Work out the finished part from the listing and answer in its coordinate system (mm). A direction names the side the tool comes from. Give positions to 0.01 mm unless a question says otherwise; leave off trailing zeros. Order: outer loops, then holes, each group sorted by start corner. A loop starts at its lowest first (then second) coordinate and runs counter-clockwise, first axis right, second up. Notation, with made-up numbers: M 67.5,-11.5 L 105.5,-11.5 A6 ccw 105.5,-7.5 Z; hole C 74,75.25 d4. An arc over 180 degrees is marked long. One line per item, written item: value.
from build123d import *

# Parameters (mm, degrees)
F0_R          = 18.15
F0_R_2        = 18.902714
F1_DEPTH      = 76.2
F2_R          = 15.292953
F3_DEPTH      = 38.1
F3_DEPTH_BACK = 38.1


with BuildPart() as f1:
    # F0 (on Front) → F1 (new body)
    with BuildSketch(Plane.XZ):
        with BuildLine():
            Line((35.557076, -57.612903), (35.557076, 57.612903))
            ThreePointArc((35.557076, 57.612903), (0, 93.16998), (-35.557076, 57.612903))
            Line((-35.557076, 57.612903), (-35.557076, -57.612903))
            ThreePointArc((-35.557076, -57.612903), (0, -93.16998), (35.557076, -57.612903))
        make_face()
        with Locations((0, -57.612903)):
            Circle(F0_R, mode=Mode.SUBTRACT)
        with Locations((0, 57.612903)):
            Circle(F0_R_2, mode=Mode.SUBTRACT)
    extrude(amount=F1_DEPTH)

    # F2 (on Top) → F3 (join, two sides)
    with BuildSketch(Plane.XY) as f3_sk:
        with BuildLine():
            ThreePointArc((-26.573732, 52.381215), (0, 31.492677), (26.573732, 52.381215))
            ThreePointArc((26.573732, 52.381215), (27.153292, 55.587559), (27.347397, 58.840074))
            ThreePointArc((27.347397, 58.840074), (-3.252515, 85.993366), (-26.573732, 52.381215))
        make_face()
        with Locations((0, 58.840074)):
            Circle(F2_R, mode=Mode.SUBTRACT)
        with BuildLine():
            Line((26.573732, 0), (26.573732, 52.381215))
            ThreePointArc((26.573732, 52.381215), (0, 31.492677), (-26.573732, 52.381215))
            Line((-26.573732, 52.381215), (-26.573732, 0))
            Line((-26.573732, 0), (26.573732, 0))
        make_face()
    extrude(amount=F3_DEPTH)
    extrude(f3_sk.sketch, amount=-F3_DEPTH_BACK)


solid = f1.part
(1) Find the intervals of material crossed by probe 1 along Z at (x, y) = (0, -33); probe 2 along Z at (x, y) = (12.5, -5.5); probe 3 along X at (y, z) = (38.5, -13), in increasing order. Write a range as from..to.
Findings:
probe 1: z = -93.17..-75.76, -39.46..38.71, 76.52..93.17
probe 2: z = -90.9..-70.77, -44.45..43.43, 71.79..90.9
probe 3: x = -26.57..26.57
(2) Which of the six approach directions +Z, -Z, +X, -X, +Y, -Y give full straight-line access (tool end or side, diameter ignored) to faces 4 (the flat face through (0, 34, -38.1)), 5 (the flat face through (0, 34, 38.1)), 6 (the flat face through (-35.557, -38, 1)), 7 (the flat face through (26.574, 26, 1)), 8 (the flat face through (-26.574, 27, 1))?
Findings:
face 4: -Z, +X, -X, +Y
face 5: +Z, +X, -X, +Y
face 6: +Z, -Z, -X, +Y, -Y
face 7: +Z, -Z, +X
face 8: +Z, -Z, -X
(3) Section C-C, the plane y = -51 is taken. Give the vertices of the cut face in (x, z), then the cut area to 3 significant figures.
Findings:
outline: M -35.56,-57.61 A35.56 ccw 35.56,-57.61 L 35.56,57.61 A35.56 ccw -35.56,57.61 Z; hole C 0,57.61 d37.81; hole C 0,-57.61 d36.3
area: 10,000 mm^2
(4) Section A-A, the plane x = 0 is taken. Give the vertices of the cut face in (y, z).
Findings:
outline: M -76.2,-93.17 L 0,-93.17 L 0,-75.76 L -76.2,-75.76 Z; M -76.2,-39.46 L 0,-39.46 L 0,-38.1 L 43.55,-38.1 L 43.55,38.1 L 0,38.1 L 0,38.71 L -76.2,38.71 Z; M -76.2,76.52 L 0,76.52 L 0,93.17 L -76.2,93.17 Z; M 74.13,-38.1 L 86.19,-38.1 L 86.19,38.1 L 74.13,38.1 Z
(5) Section B-B, the plane z = -23 is taken. Give the vertices of the cut face in (x, y), then the cut area to 3 significant figures.
Findings:
outline: M -35.56,-76.2 L 35.56,-76.2 L 35.56,0 L 26.57,0 L 26.57,52.38 A27.35 ccw 27.35,58.84 A27.35 ccw long -26.57,52.38 L -26.57,0 L -35.56,0 Z; hole C 0,58.84 d30.59
area: 8,990 mm^2
(6) Determine the mould class of faces 1 (the cylindrical face through (-3.935, -37.567, -75.331)), 2 (the cylindrical face through (8.221, 71.735, -0.533)), 3 (the flat face through (0, -76.2, 1)) for opening direction Y: pulls with the +Y half, pulls with the -Y half, needs draft (parallel to the pull), parting line crosses it, or undercut.
Findings:
face 1: needs draft
face 2: undercut
face 3: pulls with the -Y half
(7) Section D-D, the plane y = 3 is taken. Give the vertices of the cut face in (x, z), then the cut area to 3 significant figures.
Findings:
outline: M -26.57,-38.1 L 26.57,-38.1 L 26.57,38.1 L -26.57,38.1 Z
area: 4,050 mm^2
(8) Given P1, Ø21.5, axis at x = 13.5, z = -33.5, coming from the +Y side; P2, Ø10, axis at x = -20, z = -24, coming from the +Y side; P3, Ø6, axis at y = 11.5, z = -27, coming from the -X side; P4, Ø6, axis at x = 8, z = 45, coming from the +Y side, each flat-ended and moving along its own axis, determine where each tip first touches the part or whether it passes through.
Findings:
P1: stops at y = 86.05
P2: stops at y = 81.71
P3: stops at x = -26.57
P4: passes through
